```python
from build123d import *

# Parameters (mm, degrees)
SKETCH1_R           = 609.6
BOSS_EXTRUDE1_DEPTH = 12.7
SKETCH2_R           = 11
CUT_EXTRUDE1_DEPTH  = 12.7


with BuildPart() as part:
    # Sketch1 → Boss-Extrude1 (new body)
    with BuildSketch(Plane.XY):
        Circle(SKETCH1_R)
    extrude(amount=BOSS_EXTRUDE1_DEPTH)

    # Sketch2 → Cut-Extrude1 (cut)
    with BuildSketch(Plane.XY):
        with Locations((0, 558.8)):
            Circle(SKETCH2_R)
        with Locations((279.4, 483.934995635)):
            Circle(SKETCH2_R)
        with Locations((483.934995635, 279.4)):
            Circle(SKETCH2_R)
        with Locations((558.8, 0)):
            Circle(SKETCH2_R)
        with Locations((483.934995635, -279.4)):
            Circle(SKETCH2_R)
        with Locations((279.4, -483.934995635)):
            Circle(SKETCH2_R)
        with Locations((0, -558.8)):
            Circle(SKETCH2_R)
        with Locations((-279.4, -483.934995635)):
            Circle(SKETCH2_R)
        with Locations((-483.934995635, -279.4)):
            Circle(SKETCH2_R)
        with Locations((-558.8, 0)):
            Circle(SKETCH2_R)
        with Locations((-483.934995635, 279.4)):
            Circle(SKETCH2_R)
        with Locations((-279.4, 483.934995635)):
            Circle(SKETCH2_R)
    extrude(amount=CUT_EXTRUDE1_DEPTH, mode=Mode.SUBTRACT)


solid = part.part
```
Read the model definition and answer for the solid it produces. Units are mm, in the model's axes. Coordinates: 2 decimals unless noted, no trailing zeros. Write each loop counter-clockwise with the first axis right and the second up, starting at its lowest first coordinate (ties: lowest second). Pieces come first, ordered by that corner, then holes. Notation, with made-up numbers: (13.5, -35) - (41.5, -35) arc R20 ccw to (41.5, -1) - close; hole circle Ø2 at (-13.5, 33.25). An arc over 180 degrees is marked (long way). Answer as a JSON object with one key per item and string values. Group by question number.
1. Each of these flat-tipped pins is pushed along its axis until it touches: P1, Ø5, axis at y = 229, z = 7, coming from the +X side; P2, Ø3, axis at x = 196.5, z = 2, coming from the -Y side. Where does it stop, or does it pass through?
2. Consider L1, parallel to Y at x = 0, z = 2.5; L2, parallel to Y at x = 279.4, z = 2.5 (3 decimals); L3, parallel to X at y = -559.5, z = 1.5. Determine where each line is inside the solid, lowest interval first. Write a range as [from, to].
3. A cutting plane is placed at A-A (z = 9). Give the number of separate pieces and of enclosed holes in the cut face, plus the area to 3 significant figures.
4. A cutting plane is placed at C-C (x = 525.5). Determine the outline of the cut face in (y, z), plus the area to 3 significant figures.
5. A cutting plane is placed at B-B (y = 326). Determine the outline of the cut face in (x, z), plus the area to 3 significant figures.
Worked out:
{
 "1": {"P1": "stops at x = 565.96", "P2": "stops at y = -577.57"},
 "2": {"L1": "y = [-609.6, -569.8], [-547.8, 547.8], [569.8, 609.6]", "L2": "y = [-541.801, -494.935], [-472.935, 472.935], [494.935, 541.801]", "L3": "x = [-242.02, -10.98], [10.98, 242.02]"},
 "3": {"separate pieces": "1", "enclosed holes": "12", "area": "1,160,000 mm²"},
 "4": {"outline": "(-308.97, 0) - (308.97, 0) - (308.97, 12.7) - (-308.97, 12.7) - close", "area": "7,850 mm²"},
 "5": {"outline": "(-515.11, 0) - (515.11, 0) - (515.11, 12.7) - (-515.11, 12.7) - close", "area": "13,100 mm²"}
}
